```python
from build123d import *

# Parameters (mm, degrees)
F0_R          = 15
F1_DEPTH      = 150
F2_W          = 20
F2_H          = 20
F3_DEPTH      = 15
F3_DEPTH_BACK = 15


with BuildPart() as f1:
    # F0 (on Top) → F1 (new body)
    with BuildSketch(Plane.XY):
        Circle(F0_R)
    extrude(amount=F1_DEPTH)

    # F2 (on Right) → F3 (cut, two sides)
    with BuildSketch(Plane.YZ) as f3_sk:
        with Locations((0, 122.4774739146)):
            Rectangle(F2_W, F2_H)
    extrude(amount=-F3_DEPTH, mode=Mode.SUBTRACT)
    extrude(f3_sk.sketch, amount=F3_DEPTH_BACK, mode=Mode.SUBTRACT)


solid = f1.part
```
The listing builds one solid part. Answer for the finished solid, in the listing's coordinates (mm). A direction names the side the tool comes from. Coordinates: 2 decimals unless noted, no trailing zeros. Loops run counter-clockwise (first coordinate to the right, second up) from the corner with the lowest first, then second, coordinate; pieces in that order, holes last. Notation, with made-up numbers: (-5.75, 66) - (31.25, 66) arc R19 ccw to (31.25, 75) - close; hole circle Ø10 at (64, 11). An arc over 180 degrees is marked (long way). Use a Markdown table: item, result. Add a question column.
1) For faces 1 (the flat face through (0, -10, 122)), 2 (the flat face through (0, 0, 0)), determine the directions among +Z, -Z, +X, -X, +Y, -Y from which every point of the face is accessible in a straight line to the end or side of a thin tool.
2) The part is cut by section A-A, the plane y = 0. Give the vertices of the cut face in (x, z), and give its area (3 significant figures).
3) The mould has two halves that part along Y. Classify faces 3 (the flat face through (0, 0, 132.477)), 4 (the cylindrical face through (-1.953, 14.872, 73.95)), 5 (the flat face through (0, 0, 150)): released by +Y, released by -Y, zero draft, split by the parting line, or undercut.
4) The part is cut by section C-C, the plane y = 7.75. Give the vertices of the cut face in (x, z), and give its area (3 significant figures).
5) The part is cut by section D-D, the plane x = -7.75. Give the vertices of the cut face in (y, z).
6) Given pin 1 (12 mm diameter, centred on x = 8, z = 94.5, fed in from -Y); pin 2 (4 mm diameter, centred on y = -5.5, z = 33, fed in from +X); pin 3 (5 mm diameter, centred on x = -5, z = 119, fed in from +Y), each flat-ended and moving along its own axis, determine where each tip first touches the part or whether it passes through.
7) The part is cut by section B-B, the plane x = 0. Give the vertices of the cut face in (y, z), and give its area (3 significant figures).
8) Find the intervals of material crossed by line 1 (Z direction, x = 11, y = -7.25); line 2 (Y direction, x = 9, z = 117); line 3 (Y direction, x = -7, z = 123.5), in increasing order.
Here are the results:
| question | item | result |
|---|---|---|
| 1 | face 1 | +X, -X |
| 1 | face 2 | -Z, +X, -X, +Y, -Y |
| 2 | outline | (-15, 0) - (15, 0) - (15, 112.48) - (-15, 112.48) - close; (-15, 132.48) - (15, 132.48) - (15, 150) - (-15, 150) - close |
| 2 | area | 3,900 mm^2 |
| 3 | face 3 | undercut |
| 3 | face 4 | split by the parting line |
| 3 | face 5 | zero draft |
| 4 | outline | (-12.84, 0) - (12.84, 0) - (12.84, 112.48) - (-12.84, 112.48) - close; (-12.84, 132.48) - (12.84, 132.48) - (12.84, 150) - (-12.84, 150) - close |
| 4 | area | 3,340 mm^2 |
| 5 | outline | (-12.84, 0) - (12.84, 0) - (12.84, 150) - (-12.84, 150) - close; hole (-10, 112.48) - (10, 112.48) - (10, 132.48) - (-10, 132.48) - close |
| 6 | pin 1 | stops at y = -14.87 |
| 6 | pin 2 | stops at x = 14.59 |
| 6 | pin 3 | stops at y = 14.79 |
| 7 | outline | (-15, 0) - (15, 0) - (15, 150) - (-15, 150) - close; hole (-10, 112.48) - (10, 112.48) - (10, 132.48) - (-10, 132.48) - close |
| 7 | area | 4,100 mm^2 |
| 8 | line 1 | z = 0 to 112.48, 132.48 to 150 |
| 8 | line 2 | y = -12 to -10, 10 to 12 |
| 8 | line 3 | y = -13.27 to -10, 10 to 13.27 |
